Input: part model. Units: mm. Frame: model coordinates. Face numbers are marked on the shaded views. A direction names the side the tool comes from. Coordinates: 2 decimals unless noted, no trailing zeros. Loops run counter-clockwise (first coordinate to the right, second up) from the corner with the lowest first, then second, coordinate; pieces in that order, holes last.
Item 1: Section B-B on y = 0.75. Return loops of the section in (x, z), and give its area (3 significant figures).
Item 2: Pull-direction query (Z, two-part tool) for the marked faces 1, 2 and 3; classes: released by +Z, released by -Z, zero draft, split by the parting line, or undercut.
Item 3: Contact query for flat-ended pins moving along their axis: P1, Ø3, axis at x = -7.5, y = 4, coming from the +Z side; P2, Ø1.5, axis at x = -10, y = 4.5, coming from the -Z side; P3, Ø5, axis at x = -13, z = -5.5, coming from the +Y side. Output: stop coordinate, or through.
Item 4: Ray query, line 1 along X through (y, z) = (2.2, 0); line 2 along Z through (x, y) = (-21.5, 2.5); line 3 along Z through (x, y) = (-5, 3.25). Return the intervals inside material, ascending.
Item 5: Section C-C on x = -21. Give the number of separate pieces and of enclosed holes in the cut face, and give its area (3 significant figures).
Item 6: Reachability of the marked faces 4, 5 and 6 from +Z, -Z, +X, -X, +Y, -Y: full face, straight path, thin tool, end or side. Return the list, or none.
Item 7: Section A-A on z = 0. Return loops of the section in (x, y).
Item 8: Section D-D on z = -11. Return loops of the section in (x, y).
```python
from build123d import *

# Parameters (mm, degrees)
SKETCH1_R               = 5
BOSS_EXTRUDE1_DEPTH     = 6
FILLET1_R               = 3
SKETCH2_R               = 1.6
CUT_EXTRUDE1_DEPTH      = 36.846896658
CUT_EXTRUDE2_DEPTH      = 29.930952283
CUT_EXTRUDE2_DEPTH_BACK = 29.930952283
CUT_EXTRUDE3_DEPTH      = 29.460498942
FILLET3_R               = 1


with BuildPart() as part:
    # Sketch1 → Boss-Extrude1 (new body)
    with BuildSketch(Plane(origin=(0, 0, 0), x_dir=(1, 0, 0), z_dir=(0, 1, 0))):
        with BuildLine():
            Line((0, 8), (-17, 8))
            Line((-17, 8), (-17, 15))
            Line((-17, 15), (-24, 15))
            Line((-24, 15), (-24, -15))
            Line((-24, -15), (-17, -15))
            Line((-17, -15), (-17, -8))
            Line((-17, -8), (0, -8))
            ThreePointArc((0, -8), (8, 0), (0, 8))
        make_face()
        with Locations(Location((0, 0, 0), (0, 0, 270))):
            Circle(SKETCH1_R, mode=Mode.SUBTRACT)
    extrude(amount=BOSS_EXTRUDE1_DEPTH)

    # Fillet1
    fillet1_edges = [part.edges().sort_by_distance(p)[0] for p in [
        (-20.5, 0, -15),
        (-20.5, 6, -15),
        (-20.5, 0, 15),
        (-20.5, 6, 15),
    ]]
    fillet(fillet1_edges, radius=FILLET1_R - 0.0001)  # a hair under: the kernel refuses the full size

    # Sketch2 → Cut-Extrude1 (cut, through all)
    with BuildSketch(Plane.ZY.offset(24)):
        with Locations((-12, 3)):
            Circle(SKETCH2_R)
        with Locations((12, 3)):
            Circle(SKETCH2_R)
    extrude(amount=-CUT_EXTRUDE1_DEPTH, mode=Mode.SUBTRACT)

    # Sketch3 → Cut-Extrude2 (cut, two sides: drawn at the far end of the back side and taken through both)
    with BuildSketch(Plane.XY.offset(-CUT_EXTRUDE2_DEPTH_BACK)):
        Polygon((-17, 6), (8, 6), (8, 3), (0, 3), align=None)
    extrude(amount=CUT_EXTRUDE2_DEPTH + CUT_EXTRUDE2_DEPTH_BACK, mode=Mode.SUBTRACT)

    # Sketch4 → Cut-Extrude3 (cut, through all)
    with BuildSketch(Plane(origin=(0, 3, 0), x_dir=(1, 0, 0), z_dir=(0, 1, 0))):
        with BuildLine():
            Line((0, -6), (-16.5, -6))
            ThreePointArc((-16.5, -6), (-22.5, 0), (-16.5, 6))
            Line((-16.5, 6), (0, 6))
            ThreePointArc((0, 6), (6, 0), (0, -6))
        make_face()
    extrude(amount=CUT_EXTRUDE3_DEPTH, mode=Mode.SUBTRACT)

    # Fillet3
    fillet3_edges = [part.edges().sort_by_distance(p)[0] for p in [
        (-17, 3, -8),
        (-17, 3, 8),
    ]]
    fillet(fillet3_edges, radius=FILLET3_R)


solid = part.part
```
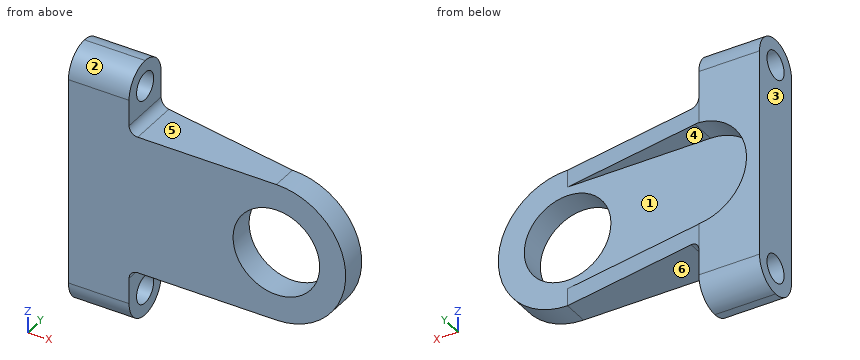
Results found:
1. outline: (-24, -13.98) - (-17, -13.98) - (-17, -9) arc R1 cw to (-16, -8) - (0, -8) arc R8 ccw to (0, 8) - (-16, 8) arc R1 cw to (-17, 9) - (-17, 13.98) - (-24, 13.98) - close; hole circle Ø10 at (0, 0)
1. area: 490 mm2
2. face 1: undercut
2. face 2: released by +Z
2. face 3: zero draft
3. P1: stops at z = 8
3. P2: stops at z = -8
3. P3: stops at y = 5.73
4. line 1: x = -24 to -5, 5 to 8
4. line 2: z = -14.96 to -13.52, -10.48 to 10.48, 13.52 to 14.96
4. line 3: z = -8 to -6, 6 to 8
5. separate pieces: 1
5. enclosed holes: 2
5. area: 132 mm2
6. face 4: +X, +Y
6. face 5: +Z, +X, +Y, -Y
6. face 6: -Z, +X, +Y, -Y
7. outline: (-24, 0) - (-5, 0) - (-5, 3) - (-22.5, 3) - (-22.5, 6) - (-24, 6) - close; (5, 0) - (8, 0) - (8, 3) - (5, 3) - close
8. outline: (-24, 0) - (-17, 0) - (-17, 1.75) - (-24, 1.75) - close; (-24, 4.25) - (-17, 4.25) - (-17, 6) - (-24, 6) - close
